Here's how the part is built. I have some questions about the finished solid (model axes, mm). Face numbers are marked on the shaded views. A direction names the side the tool comes from. Give positions to 0.01 mm unless a question says otherwise; leave off trailing zeros. Write each loop counter-clockwise with the first axis right and the second up, starting at its lowest first coordinate (ties: lowest second). Pieces come first, ordered by that corner, then holes. Notation, with made-up numbers: (-39.5, 59) - (-13.5, 59) arc R26 ccw to (-13.5, 97) - close; hole circle Ø10 at (-6.5, 31.5). An arc over 180 degrees is marked (long way). One line per item, written item: value. Start each with the question number.
1) Imagine slicing it at D-D on z = 22. Count the separate pieces of the cut face and the enclosed holes in it, plus the area to 3 significant figures.
2) Imagine slicing it at A-A on y = 84.5. Write out the boundary of the cut face in (x, z).
3) Imagine slicing it at B-B on x = -136. Write out the boundary of the cut face in (y, z) (3 decimals).
4) We'd pull the mould along Y, two halves only. Please class the marked faces 6, 7, 8 and 9: +Y half, -Y half, draft (parallel to the pull), parting line (faces both ways), or undercut.
5) I'm going to push flat-ended pins straight in: P1, Ø3, axis at x = -152, z = 23, coming from the +Y side; P2, Ø4, axis at y = 37.5, z = 4.5, coming from the +X side; P3, Ø5, axis at x = -117.5, y = -51, coming from the -Z side; P4, Ø24, axis at y = 132, z = 45, coming from the +X side. Where does each tip first touch, or does it pass through?
6) Imagine slicing it at C-C on x = -269.5. Write out the boundary of the cut face in (y, z) (3 decimals).
7) On a 3-axis mill with a long thin cutter (end or side, diameter ignored), from which of +Z, -Z, +X, -X, +Y, -Y can I reach the whole of each face in a straight line? I mean the marked faces 1, 2, 3, 4 and 5. Say none if no direction works.
8) Please list where these lines run through material, in increasing order: L1, parallel to Y at x = -396, z = 9.5; L2, parallel to Y at x = 147, z = 67; L3, parallel to X at y = 142.5, z = 6. Write a range as [from, to].
from build123d import *

# Parameters (mm, degrees)
F1_DEPTH  = 90
F3_DEPTH  = 80
F14_W     = 60.7640445232
F14_H     = 85.0984491408
F14_W_2   = 67.515194416
F14_H_2   = 10.8465999365
F15_DEPTH = 25
F16_W     = 49.2283031344
F16_H     = 38.4706258774
F17_DEPTH = 25
F18_W     = 81.171695143
F18_H     = 78.6929726601
F18_W_2   = 13.7816295028
F18_H_2   = 67.5387531519
F19_DEPTH = 25
F20_W     = 44.0124189481
F20_H     = 9.0348646045
F21_DEPTH = 70
F22_W     = 52.3186028004
F22_H     = 8.4803402424
F23_DEPTH = 25
F24_T     = -2.5


# Not quite as in the source:
# - a shell that OpenCascade refuses in one call is made with other operations: the cavity is built on its own and cut out
# - the program builds the solid bodies; features that only make, move or delete a surface that nothing else refers to are left out


with BuildPart() as f1:
    # F0 (on Top) → F1 (new body)
    with BuildSketch(Plane.XY):
        Polygon((0, -103.756165579), (61.2453594729, -103.756165579), (209.3763612108, -103.756165579), (209.3763612108, -63.756165579), (84.9471986294, -63.756165579), (84.9471986294, 48.3620613813), (72.6846382022, 48.3620613813), (72.6846382022, 208.6838036776), (-109.8914146423, 208.6838036776), (-109.8914146423, 48.3620613813), (-190.279379487, 48.3620613813), (-190.279379487, 152.8209894896), (-315.6301081181, 152.8209894896), (-315.6301081181, 48.3620613813), (-337.8433585167, 48.3620613813), (-337.8433585167, 29.8324227333), (-464.4817113876, 29.8324227333), (-464.4817113876, -156.8707674742), (-337.8433585167, -156.8707674742), (-337.8433585167, -195.1335072517), (-440.5674934387, -195.1335072517), (-440.5674934387, -233.3962619305), (-337.8433585167, -233.3962619305), (-337.8433585167, -257.3104500771), (0, -257.3104500771), align=None)
    extrude(amount=F1_DEPTH)

    # F2 (on face) → F3 (cut)
    with BuildSketch(Plane.XY.offset(90)):
        Polygon((-334.4984054565, 27.9887765646), (-462.5793099403, 27.9887765646), (-462.5793099403, -152.908667922), (-334.4984054565, -152.908667922), (-334.4984054565, -198.7856328487), (-435.5817735195, -198.7856328487), (-435.5817735195, -229.2267084122), (-334.4984054565, -229.2267084122), (-334.4984054565, -253.2849907875), (-6.9517553784, -253.2849907875), (-6.9517553784, -96.1697399616), (204.1718363762, -96.1697399616), (204.1718363762, -67.2016069293), (80.44359833, -67.2016069293), (80.44359833, 43.2700514793), (65.7140463591, 43.2700514793), (65.7140463591, 201.8582522869), (-104.6577990055, 201.8582522869), (-104.6577990055, 43.2700552046), (-194.9990689754, 43.2700552046), (-194.9990689754, 147.8498876095), (-311.8534982204, 147.8498876095), (-311.8534982204, 44.2520268261), (-334.4984054565, 44.2520268261), align=None)
    extrude(amount=-F3_DEPTH, mode=Mode.SUBTRACT)

    # F14 (on face) → F15 (join)
    with BuildSketch(Plane.XY.offset(10)):
        with Locations((-394.2892104387, -14.5604480058)):
            Rectangle(F14_W, F14_H)
        with Locations((-401.1757969856, -147.4853679538)):
            Rectangle(F14_W_2, F14_H_2)
    extrude(amount=F15_DEPTH)

    # F16 (on face) → F17 (cut)
    with BuildSketch(Plane.YZ.offset(-462.5793099403)):
        with Locations((-69.2342929542, 59.7355216742)):
            Rectangle(F16_W, F16_H)
    extrude(amount=-F17_DEPTH, mode=Mode.SUBTRACT)

    # F18 (on face) → F19 (join)
    with BuildSketch(Plane.XY.offset(10)):
        with Locations((-20.1654676348, 162.5117659569)):
            Rectangle(F18_W, F18_H)
        with Locations((-97.7669842541, 152.3723676801)):
            Rectangle(F18_W_2, F18_H_2)
    extrude(amount=F19_DEPTH)

    # F20 (on face) → F21 (join)
    with BuildSketch(Plane.XY.offset(10)):
        with Locations((31.1586786993, -91.6523076594)):
            Rectangle(F20_W, F20_H)
    extrude(amount=F21_DEPTH)

    # F22 (on face) → F23 (join)
    with BuildSketch(Plane.XY.offset(10)):
        with Locations((117.6677644253, -91.9295698404)):
            Rectangle(F22_W, F22_H)
    extrude(amount=F23_DEPTH)

    # F24: a shell. OpenCascade refuses it in one call, so the cavity is built on its own and cut out:
    # the body offset inwards by the wall thickness, plus a prism from it out through each open face.
    f24_core = offset(f1.part, amount=F24_T, kind=Kind.INTERSECTION, mode=Mode.PRIVATE)
    f24_exits = [f24_core.faces().sort_by_distance(p)[0] for p in [
        (31.158679, -89.634875, 42.5),
    ]]
    add(f24_core, mode=Mode.SUBTRACT)
    extrude(f24_exits, amount=-F24_T, mode=Mode.SUBTRACT)


solid = f1.part
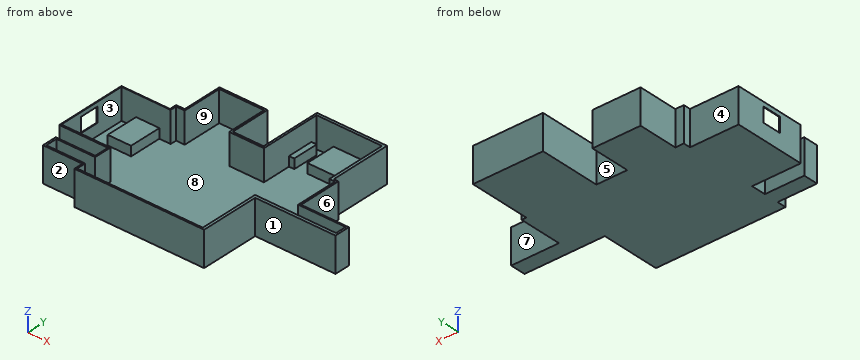
Numbers:
1. separate pieces: 1
1. enclosed holes: 4
1. area: 12,300 mm^2
2. outline: (-315.63, 0) - (-190.28, 0) - (-190.28, 90) - (-195, 90) - (-195, 10) - (-311.85, 10) - (-311.85, 90) - (-315.63, 90) - close; (-109.89, 0) - (72.68, 0) - (72.68, 90) - (65.71, 90) - (65.71, 10) - (-104.66, 10) - (-104.66, 90) - (-109.89, 90) - close; hole (-313.13, 2.5) - (-192.78, 2.5) - (-192.78, 7.5) - (-313.13, 7.5) - close; hole (-107.39, 2.5) - (70.18, 2.5) - (70.18, 87.5) - (68.21, 87.5) - (68.21, 7.5) - (-107.16, 7.5) - (-107.16, 87.5) - (-107.39, 87.5) - close
3. outline: (-257.31, 0) - (48.362, 0) - (48.362, 90) - (43.27, 90) - (43.27, 10) - (-253.285, 10) - (-253.285, 90) - (-257.31, 90) - close; hole (-254.81, 2.5) - (45.862, 2.5) - (45.862, 87.5) - (45.77, 87.5) - (45.77, 7.5) - (-254.81, 7.5) - close
4. face 6: draft
4. face 7: +Y half
4. face 8: undercut
4. face 9: undercut
5. P1: y = 48.36
5. P2: x = 84.95
5. P3: z = 0
5. P4: x = 72.68
6. outline: (-257.31, 0) - (152.821, 0) - (152.821, 90) - (147.85, 90) - (147.85, 10) - (-253.285, 10) - (-253.285, 90) - (-257.31, 90) - close; hole (-254.81, 2.5) - (150.321, 2.5) - (150.321, 7.5) - (-254.81, 7.5) - close
7. face 1: +Z, -Z, +X, -Y
7. face 2: +Z, -Z, -X, -Y
7. face 3: +Z
7. face 4: +Z, -Z, -X, +Y
7. face 5: +Z, -Z, +Y
8. L1: [-233.4, -195.13], [-156.87, -154.37], [-144.56, -54.61], [27.33, 29.83]
8. L2: [-103.76, -101.26], [-98.67, -96.17], [-67.2, -63.76]
8. L3: [-315.63, -313.13], [-192.78, -190.28], [-109.89, -107.39], [70.18, 72.68]
